```python
from build123d import *

# Parameters (mm, degrees)
BOSS_EXTRUDE1_DEPTH = 2
SKETCH3_R           = 8.2
CUT_EXTRUDE2_DEPTH  = 43.547600128
SKETCH4_R           = 1.5
SKETCH4_R_2         = 1.618660888
SKETCH4_R_3         = 1.441296675
CUT_EXTRUDE3_DEPTH  = 43.547600128
SKETCH6_W           = 20
SKETCH6_H           = 2
BOSS_EXTRUDE2_DEPTH = 12
FILLET1_R           = 3
FILLET2_R           = 3
SKETCH7_R           = 1.5
CUT_EXTRUDE4_DEPTH  = 54.930795553
FILLET3_R           = 3


with BuildPart() as part:
    # Sketch1 → Boss-Extrude1 (new body)
    with BuildSketch(Plane.XY):
        with BuildLine():
            Line((-19.779193206, 13.552016985), (24.220806794, 13.552016985))
            ThreePointArc((24.220806794, 13.552016985), (25.635020356, 12.966230548), (26.220806794, 11.552016985))
            Line((26.220806794, 11.552016985), (26.220806794, -6.447983015))
            ThreePointArc((26.220806794, -6.447983015), (25.635020356, -7.862196577), (24.220806794, -8.447983015))
            Line((24.220806794, -8.447983015), (17.220806794, -8.447983015))
            ThreePointArc((17.220806794, -8.447983015), (13.685272888, -9.912449109), (12.220806794, -13.447983015))
            Line((12.220806794, -13.447983015), (12.220806794, -33.447983015))
            Line((12.220806794, -33.447983015), (-7.779193206, -33.447983015))
            Line((-7.779193206, -33.447983015), (-7.779193206, -13.447983015))
            ThreePointArc((-7.779193206, -13.447983015), (-9.2436593, -9.912449109), (-12.779193206, -8.447983015))
            Line((-12.779193206, -8.447983015), (-19.779193206, -8.447983015))
            ThreePointArc((-19.779193206, -8.447983015), (-21.193406768, -7.862196577), (-21.779193206, -6.447983015))
            Line((-21.779193206, -6.447983015), (-21.779193206, 11.552016985))
            ThreePointArc((-21.779193206, 11.552016985), (-21.193406768, 12.966230548), (-19.779193206, 13.552016985))
        make_face()
    extrude(amount=BOSS_EXTRUDE1_DEPTH)

    # Sketch3 → Cut-Extrude2 (cut, through all)
    with BuildSketch(Plane.XY.offset(2)):
        with Locations((-10.929193206, 1.702016985)):
            Circle(SKETCH3_R)
        with Locations((15.370806794, 1.702016985)):
            Circle(SKETCH3_R)
    extrude(amount=-CUT_EXTRUDE2_DEPTH, mode=Mode.SUBTRACT)

    # Sketch4 → Cut-Extrude3 (cut, through all)
    with BuildSketch(Plane.XY.offset(2)):
        with Locations((-19.079193206, 11.252016985)):
            Circle(SKETCH4_R)
        with Locations((-19.279193206, -6.247983015)):
            Circle(SKETCH4_R_2)
        with Locations((23.520806794, 11.252016985)):
            Circle(SKETCH4_R_3)
        with Locations((23.520806794, -6.247983015)):
            Circle(SKETCH4_R)
    extrude(amount=-CUT_EXTRUDE3_DEPTH, mode=Mode.SUBTRACT)

    # Sketch6 → Boss-Extrude2 (add)
    with BuildSketch(Plane.XY.offset(2)):
        with Locations((2.220806794, -32.447983015)):
            Rectangle(SKETCH6_W, SKETCH6_H)
    extrude(amount=BOSS_EXTRUDE2_DEPTH)

    # Fillet1
    fillet1_edges = [part.edges().sort_by_distance(p)[0] for p in [
        (2.220806794, -33.447983015, 0),
    ]]
    fillet(fillet1_edges, radius=FILLET1_R)

    # Fillet2
    fillet2_edges = [part.edges().sort_by_distance(p)[0] for p in [
        (2.220806794, -31.447983015, 2),
    ]]
    fillet(fillet2_edges, radius=FILLET2_R)

    # Sketch7 → Cut-Extrude4 (cut, through all)
    with BuildSketch(Plane(origin=(0, -31.447983015, 0), x_dir=(1, 0, 0), z_dir=(0, 1, 0))):
        with Locations(Location((-4.279193206, -9.5, 0), (0, 0, 270))):
            Circle(SKETCH7_R)
        with Locations(Location((7.720806794, -9.5, 0), (0, 0, 270))):
            Circle(SKETCH7_R)
    extrude(amount=-CUT_EXTRUDE4_DEPTH, mode=Mode.SUBTRACT)

    # Fillet3
    fillet3_edges = [part.edges().sort_by_distance(p)[0] for p in [
        (-7.779193206, -32.447983015, 14),
        (12.220806794, -32.447983015, 14),
    ]]
    fillet(fillet3_edges, radius=FILLET3_R)


solid = part.part
```
Part model, mm, in its own coordinate system. A direction names the side the tool comes from. Give positions to 0.01 mm unless a question says otherwise; leave off trailing zeros. Write each loop counter-clockwise with the first axis right and the second up, starting at its lowest first coordinate (ties: lowest second). Pieces come first, ordered by that corner, then holes. Notation, with made-up numbers: (3.5, -33.75) -> (27.5, -33.75) arc R12 ccw to (27.5, -12.75) -> close; hole circle Ø9 at (-11.75, -19.75). An arc over 180 degrees is marked (long way). Put each result on its own line as item: value. Start each with the question number.
Item 1: Wall check: L1, parallel to X at y = -31.9, z = 9.5; L2, parallel to Y at x = -2.5, z = 12.75; L3, parallel to Z at x = 5, y = -1. Give the ranges that are in metal, low to high. Write a range as [from, to].
Item 2: Cut at B-B (x = 13.5). List the corners of the cut face in (y, z).
Item 3: Pin check, flat tips, straight feed: pin 1 Ø2 at (x, z) = (4.5, 10) entering from +Y; pin 2 Ø21 at (x, y) = (-7, -7) entering from +Z; pin 3 Ø4 at (x, y) = (4.5, 5) entering from -Z; pin 4 Ø0.6 at (x, z) = (21.5, 1) entering from -Y. Stop position of each tip, or through.
Item 4: Cut at D-D (x = -12). List the corners of the cut face in (y, z), then the cut area to 3 significant figures.
Item 5: Which spindle directions (+Z, -Z, +X, -X, +Y, -Y) get a long thin tool onto all of the face, cutting with end or side? Do faces 4 (the face through (12.221, -26.5, 1.8)), 5 (the face through (-9.205, -9.952, 0.986)). Say none if no direction does.
Item 6: Cut at A-A (z = 9.5). List the corners of the cut face in (x, y), then the cut area to 3 significant figures.
Item 7: Cut at C-C (z = 6.25). List the corners of the cut face in (x, y), then the cut area to 3 significant figures.
Item 8: Pull direction Y, two halves, no side cores. Call faces 1 (the face through (3, -2, 2)), 2 (the face through (2, -31.448, 9)), 3 (the face through (-12, 9.83, 1.01)): pulls with the +Y half, pulls with the -Y half, needs draft (parallel to the pull), parting line crosses it, or undercut.
Answer list:
1. L1: x = [-7.78, -5.78], [-2.78, 6.22], [9.22, 12.22]
1. L2: y = [-33.45, -31.45]
1. L3: z = [0, 2]
2. outline: (-10.11, 0) -> (-6.28, 0) -> (-6.28, 2) -> (-10.11, 2) -> close; (9.69, 0) -> (13.55, 0) -> (13.55, 2) -> (9.69, 2) -> close
3. pin 1: stops at y = -31.45
3. pin 2: stops at z = 2
3. pin 3: stops at z = 0
3. pin 4: stops at y = -8.45
4. outline: (-8.51, 0) -> (-6.43, 0) -> (-6.43, 2) -> (-8.51, 2) -> close; (9.83, 0) -> (13.55, 0) -> (13.55, 2) -> (9.83, 2) -> close
4. area: 11.6 mm2
5. face 4: +Z, -Z, +X, -Y
5. face 5: +Z, -Z, -X, -Y
6. outline: (-7.78, -33.45) -> (-5.78, -33.45) -> (-5.78, -31.45) -> (-7.78, -31.45) -> close; (-2.78, -33.45) -> (6.22, -33.45) -> (6.22, -31.45) -> (-2.78, -31.45) -> close; (9.22, -33.45) -> (12.22, -33.45) -> (12.22, -31.45) -> (9.22, -31.45) -> close
6. area: 28.0 mm2
7. outline: (-7.78, -33.45) -> (12.22, -33.45) -> (12.22, -31.45) -> (-7.78, -31.45) -> close
7. area: 40.0 mm2
8. face 1: needs draft
8. face 2: pulls with the +Y half
8. face 3: undercut
